from build123d import *

# Parameters (mm, degrees)
F0_R          = 5
F1_DEPTH      = 70
F1_DEPTH_BACK = 45
F2_R          = 4
F3_DEPTH      = 7
F4_R          = 3.25
F5_DEPTH      = 3
F6_R          = 2
F7_DEPTH      = 3.54
F8_R          = 1
F9_DEPTH      = 3.8


with BuildPart() as f1:
    # F0 (on Top) → F1 (new body, two sides)
    with BuildSketch(Plane.XY) as f1_sk:
        Circle(F0_R)
    extrude(amount=F1_DEPTH)
    extrude(f1_sk.sketch, amount=-F1_DEPTH_BACK)

    # F2 (on face) → F3 (join)
    with BuildSketch(Plane(origin=(0, 0, -45), x_dir=(1, 0, 0), z_dir=(0, 0, -1))):
        Circle(F2_R)
    extrude(amount=F3_DEPTH)

    # F4 (on face) → F5 (join)
    with BuildSketch(Plane(origin=(0, 0, -52), x_dir=(1, 0, 0), z_dir=(0, 0, -1))):
        Circle(F4_R)
    extrude(amount=F5_DEPTH)

    # F6 (on face) → F7 (join)
    with BuildSketch(Plane(origin=(0, 0, -55), x_dir=(1, 0, 0), z_dir=(0, 0, -1))):
        Circle(F6_R)
    extrude(amount=F7_DEPTH)

    # F8 (on face) → F9 (join)
    with BuildSketch(Plane(origin=(0, 0, -58.54), x_dir=(1, 0, 0), z_dir=(0, 0, -1))):
        Circle(F8_R)
    extrude(amount=F9_DEPTH)


solid = f1.part
Verification items for the finished model (mm, model axes). A direction names the side the tool comes from. Give positions to 0.01 mm unless a question says otherwise; leave off trailing zeros. Order: outer loops, then holes, each group sorted by start corner. A loop starts at its lowest first (then second) coordinate and runs counter-clockwise, first axis right, second up. Notation, with made-up numbers: (0, 32.25) -> (5, 32.25) arc R15 ccw to (5, 57.25) -> close; hole circle Ø4 at (16.5, 79.25). An arc over 180 degrees is marked (long way). Answer as CSV lines item,"result".
Q1. Sectioned sample at B-B on z = -49. Record the cut outline in (x, y).
Solutions:
outline,"circle Ø8 at (0, 0)"
Q2. Access from +Z, -Z, +X, -X, +Y, -Y to the whole of each face (thin tool, end or side, straight path). Record for faces 1 (the cylindrical face through (-0.867, 3.905, -48.451)), 2 (the flat face through (0, 0, -62.34)).
Solutions:
face 1,"-Z"
face 2,"-Z, +X, -X, +Y, -Y"
Q3. Sectioned sample at A-A on z = -17. Record the cut outline in (x, y), plus the area to 3 significant figures.
Solutions:
outline,"circle Ø10 at (0, 0)"
area,"78.5 mm²"
Q4. Depth check by flat-ended pin: pin 1 (2 mm diameter, centred on y = 3, z = 35.5, fed in from -X); pin 2 (4 mm diameter, centred on x = -3, y = 1.5, fed in from -Z); pin 3 (2 mm diameter, centred on x = 0.5, y = -1, fed in from -Z); pin 4 (3 mm diameter, centred on y = 1, z = -48.5, fed in from +X). Enter the tip coordinate at first touch or a pass-through.
Solutions:
pin 1,"stops at x = -4.58"
pin 2,"stops at z = -58.54"
pin 3,"stops at z = -62.34"
pin 4,"stops at x = 4"
Q5. Scan lines: probe 1 along Z at (x, y) = (1, 4); probe 2 along Z at (x, y) = (-1.5, -1.5); probe 3 along Y at (x, z) = (-0.25, 27.5). Record each from-to range of solid material in increasing order.
Solutions:
probe 1,"z = -45 to 70"
probe 2,"z = -55 to 70"
probe 3,"y = -4.99 to 4.99"
